from build123d import *

# Parameters (mm, degrees)
BOSS_EXTRUDE1_DEPTH = 8
SKETCH3_R           = 1.5
CUT_EXTRUDE1_DEPTH  = 6.2
FILLET4_R           = 2
FILLET5_R           = 2


with BuildPart() as part:
    # Sketch2 → Boss-Extrude1 (new body)
    with BuildSketch(Plane(origin=(0, 0, 0), x_dir=(1, 0, 0), z_dir=(0, 1, 0))):
        with BuildLine():
            ThreePointArc((0, 10), (-10, 0), (0, -10))
            add(Edge.make_bspline(
                [(0, -10), (22.676468469, -10), (45.303936393, -8), (68, -8)],
                knots=[0, 0, 0, 0, 1, 1, 1, 1], degree=3))
            ThreePointArc((68, -8), (76, 0), (68, 8))
            add(Edge.make_bspline(
                [(0, 10), (22.676468469, 10), (45.303936393, 8), (68, 8)],
                knots=[0, 0, 0, 0, 1, 1, 1, 1], degree=3))
        make_face()
    extrude(amount=BOSS_EXTRUDE1_DEPTH)

    # Sketch3 → Cut-Extrude1 (cut)
    with BuildSketch(Plane(origin=(0, 8, 0), x_dir=(1, 0, 0), z_dir=(0, 1, 0))):
        with Locations(Location((0, 0, 0), (0, 0, 270))):
            Circle(SKETCH3_R)
        with Locations(Location((68, 0, 0), (0, 0, 270))):
            Circle(SKETCH3_R)
        with Locations(Location((20, 0, 0), (0, 0, 270))):
            Circle(SKETCH3_R)
        with Locations(Location((24, 0, 0), (0, 0, 270))):
            Circle(SKETCH3_R)
        with Locations(Location((60, 0, 0), (0, 0, 270))):
            Circle(SKETCH3_R)
        with Locations(Location((52, 0, 0), (0, 0, 270))):
            Circle(SKETCH3_R)
        with Locations(Location((44, 0, 0), (0, 0, 270))):
            Circle(SKETCH3_R)
    extrude(amount=-CUT_EXTRUDE1_DEPTH, mode=Mode.SUBTRACT)

    # Fillet4
    fillet4_edges = [part.edges().sort_by_distance(p)[0] for p in [
        (33.999990473, 8, 8.999676096),
        (76, 8, 0),
        (33.999990473, 8, -8.999676096),
        (-10, 8, 0),
    ]]
    fillet(fillet4_edges, radius=FILLET4_R)

    # Fillet5
    fillet5_edges = [part.edges().sort_by_distance(p)[0] for p in [
        (76, 0, 0),
        (33.999990473, 0, 8.999676096),
        (-10, 0, 0),
        (33.999990473, 0, -8.999676096),
    ]]
    fillet(fillet5_edges, radius=FILLET5_R)


solid = part.part
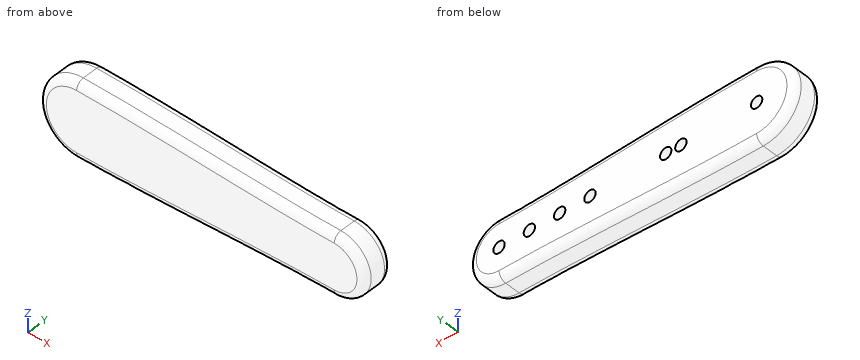
Geometry: final body of the model. Coordinates: model frame, mm. Give positions to 0.01 mm unless a question says otherwise; leave off trailing zeros. Put each result on its own line as item: value.
1. Cut plane A-A (y = 4.75). Count the separate pieces of the cut face and the enclosed holes in it, plus the area to 3 significant figures.
Taken from the geometry:
separate pieces: 1
enclosed holes: 7
area: 1,430 mm2
2. Ray query, line 1 along Y through (x, z) = (69, 1); line 2 along Z through (x, y) = (61, 1.5); line 3 along Z through (x, y) = (17.5, 1.5). Return the intervals inside material, ascending. Write a range as [from, to].
Taken from the geometry:
line 1: y = [0, 1.8]
line 2: z = [-8, 8]
line 3: z = [-9.61, 9.61]
3. Pin query (flat end, axial travel): P1, Ø5, axis at x = 68, z = 0, coming from the -Y side; P2, Ø2.5, axis at x = 0, z = 0, coming from the +Y side; P3, Ø3, axis at x = 43, y = 6.5, coming from the -Z side; P4, Ø3, axis at x = 12.5, y = 1, coming from the +Z side. Return the tip coordinate at first contact, or that it passes through.
Taken from the geometry:
P1: stops at y = 0
P2: stops at y = 1.8
P3: stops at z = -8.67
P4: stops at z = 9.85
